Model file for the job. Use its own axes, mm. A direction names the side the tool comes from. Round coordinates to 2 decimals unless told otherwise and drop trailing zeros. Loops run counter-clockwise (first coordinate to the right, second up) from the corner with the lowest first, then second, coordinate; pieces in that order, holes last. Notation, with made-up numbers: M 34,38 L 85,38 A16 cw 85,68 Z; hole C 59,72 d1. An arc over 180 degrees is marked long. Use a Markdown table: item, result. Add a question column.
Q1. Cut at D-D (x = -15.5). Give the cut face in (y, z), plus the area to 3 significant figures.
Q2. Probe line 1 (Y direction, x = 15.5, z = 3.75); line 2 (Y direction, x = -15.5, z = 12); line 3 (Z direction, x = 5.5, y = 9). List the from-to ranges inside material, lowest first. Write a range as from..to.
Q3. Cut at A-A (y = -15.5). Give the cut face in (x, z).
Q4. Tool access for faces 1 (the face through (18, -19, 8)), 2 (the face through (8, 0, 15)), 3 (the face through (-9.151, -10.734, 8.381)): list every direction of +Z, -Z, +X, -X, +Y, -Y with a clear straight run to the whole face (end or side of a thin tool).
Q5. Mould opens along X. For faces 4 (the face through (13.9, 15.43, 8.38)), 5 (the face through (9, 0, 0)), 6 (the face through (-21, 15.5, 8.4)), 7 (the face through (-16.68, 14.42, 8.38)) say: +X half, -X half, draft (parallel to the pull), parting line (faces both ways), or undercut.
Q6. Cut at C-C (z = 6). Give the cut face in (x, y).
Autodesk Inventor part; units mm, degrees
ref_plane "YZ Plane" through (0, 0, 0) normal (1, 0, 0) x (0, 1, 0)
ref_plane "XZ Plane" through (0, 0, 0) normal (0, 1, 0) x (-1, 0, 0)
ref_plane "XY Plane" through (0, 0, 0) normal (0, 0, 1) x (1, 0, 0)
sketch "Sketch1" plane through (0, 0, 0) normal (0, 0, 1) x (1, 0, 0)
  line L0 (-21, 21) -> (21, 21)
  line L1 (21, 21) -> (21, -21)
  line L2 (21, -21) -> (-21, -21)
  line L3 (-21, -21) -> (-21, -15)
  arc A0 (2.3711, -6.5862) -> (2.3711, 6.5862) centre (0, 0) ccw
  line L4 (2.3711, 6.5862) -> (-21, 15)
  line L5 (-21, 15) -> (-21, 21)
  line L6 (2.3711, -6.5862) -> (-21, -15)
  line L7 (0, -29.4) -> (0, 29.4)
  line L8 (-29.4, 0) -> (29.4, 0)
  circle A1 centre (-15.5, 15.5) radius 1.6
  circle A2 centre (15.5, 15.5) radius 1.6
  circle A3 centre (15.5, -15.5) radius 1.6
  circle A4 centre (-15.5, -15.5) radius 1.6
  dimension "d0" = 21
  dimension "d1" = 21
  dimension "d2" = 21
  dimension "d3" = 21
  dimension "d4" = 7
  dimension "d5" = 15.5
  dimension "d6" = 15.5
  dimension "d7" = 15.5
  dimension "d8" = 15.5
  dimension "d9" = 15.5
  dimension "d10" = 15.5
  dimension "d11" = 15.5
  dimension "d12" = 15.5
  dimension "d13" = 3.2
  dimension "d14" = 6
extrude "Extrusion1" add sketch "Sketch1" along normal blind 17 contours L0 L7 L4 L5 | L0 L1 L8 A0 L4 L7 | L1 L2 L7 L6 A0 L8 | L7 L2 L3 L6
chamfer "Chamfer1" distance 5 angle 45 4 edges at (-21, 21, 8.5) (-21, -21, 8.5) (21, 21, 8.5) (21, -21, 8.5)
sketch "Sketch2" plane through (0, 0, 17) normal (0, 0, 1) x (1, 0, 0)
  circle A0 centre (0, 0) radius 11.2
  dimension "d20" = 22.4
extrude "Extrusion2" cut sketch "Sketch2" against normal blind 2
properties part number "motor_spacer"
Checked values:
| question | item | result |
|---|---|---|
| 1 | outline | M -21,0 L -17.1,0 L -17.1,17 L -21,17 Z; M -13.9,0 L -13.02,0 L -13.02,17 L -13.9,17 Z; M 13.02,0 L 13.9,0 L 13.9,17 L 13.02,17 Z; M 17.1,0 L 21,0 L 21,17 L 17.1,17 Z |
| 1 | area | 163 mm^2 |
| 2 | line 1 | y = -21..-17.1, -13.9..13.9, 17.1..21 |
| 2 | line 2 | y = -21..-17.1, -13.9..-13.02, 13.02..13.9, 17.1..21 |
| 2 | line 3 | z = 0..15 |
| 3 | outline | M -21,0 L -17.1,0 L -17.1,17 L -21,17 Z; M -13.9,0 L 13.9,0 L 13.9,17 L -13.9,17 Z; M 17.1,0 L 21,0 L 21,17 L 17.1,17 Z |
| 4 | face 1 | +Z, -Z, +X, -Y |
| 4 | face 2 | +Z |
| 4 | face 3 | +Z, -Z, -X |
| 5 | face 4 | undercut |
| 5 | face 5 | draft |
| 5 | face 6 | -X half |
| 5 | face 7 | undercut |
| 6 | outline | M -21,-16 L -16,-21 L 16,-21 L 21,-16 L 21,16 L 16,21 L -16,21 L -21,16 L -21,15 L 2.37,6.59 A7 cw 2.37,-6.59 L -21,-15 Z; hole C -15.5,-15.5 d3.2; hole C -15.5,15.5 d3.2; hole C 15.5,-15.5 d3.2; hole C 15.5,15.5 d3.2 |
